For this review, take the finished solid that the model builds, in its own axes (mm). Coordinates: 2 decimals unless noted, no trailing zeros. Loops run counter-clockwise (first coordinate to the right, second up) from the corner with the lowest first, then second, coordinate; pieces in that order, holes last. Notation, with made-up numbers: (12.25, 74) -> (28.25, 74) arc R31 cw to (28.25, 105) -> close; hole circle Ø4 at (-27, 39.25). An arc over 180 degrees is marked (long way). Answer in a Markdown table with one row per item.
Autodesk Inventor part; units mm, degrees
ref_plane "YZ Plane" through (0, 0, 0) normal (1, 0, 0) x (0, 1, 0)
ref_plane "XZ Plane" through (0, 0, 0) normal (0, 1, 0) x (-1, 0, 0)
ref_plane "XY Plane" through (0, 0, 0) normal (0, 0, 1) x (1, 0, 0)
sketch "Sketch1" plane through (0, 0, 0) normal (0, 0, 1) x (1, 0, 0)
  circle A0 centre (0, 0) radius 12
  circle A1 centre (-6, 6) radius 2
  circle A2 centre (-6, -6) radius 2
  circle A3 centre (6, -6) radius 2
  circle A4 centre (6, 6) radius 2
  dimension "d0" = 24
  dimension "d1" = 4
  dimension "d2" = 6
  dimension "d3" = 6
  dimension "d6" = 360
extrude "Extrusion1" add sketch "Sketch1" along normal blind 6
sketch "Sketch2" plane through (0, 0, 6) normal (0, 0, 1) x (1, 0, 0)
  circle A0 centre (0, 0) radius 3.2
  dimension "d10" = 6.4
extrude "Extrusion2" cut sketch "Sketch2" against normal through all
properties part number "MountingPiece"
Item 1: Take a section at D-D, the plane z = 1.5. State the section outline as (x, y) points.
Worked answers:
| item | result |
|---|---|
| outline | circle Ø24 at (0, 0); hole circle Ø4 at (-6, -6); hole circle Ø4 at (-6, 6); hole circle Ø6.4 at (0, 0); hole circle Ø4 at (6, -6); hole circle Ø4 at (6, 6) |
Item 2: Insertion check: pin 1 (2 mm diameter, centred on x = -3.5, z = 2, fed in from +Y); pin 2 (4.5 mm diameter, centred on x = -6, y = 6, fed in from +Z); pin 3 (2 mm diameter, centred on x = -8, z = 2, fed in from +Y). Each pin has a flat end and moves straight along its axis. Give the tip position at first contact, or say it passes through.
Worked answers:
| item | result |
|---|---|
| pin 1 | y = 11.74 |
| pin 2 | z = 6 |
| pin 3 | y = 9.75 |
Item 3: The part is to be moulded in two halves that separate along X. For faces 1 (the cylindrical face through (4.4, 7.2, 3)), 2 (the flat face through (2.5, -2.5, 0)), 3 (the cylindrical face through (-7.6, 7.2, 3)), 4 (the cylindrical face through (-11.99, -0.53, 2.96)), say which applies: +X half, -X half, draft (parallel to the pull), parting line (faces both ways), or undercut.
Worked answers:
| item | result |
|---|---|
| face 1 | undercut |
| face 2 | draft |
| face 3 | undercut |
| face 4 | parting line |
Item 4: Take a section at C-C, the plane y = 6. State the section outline as (x, z) points.
Worked answers:
| item | result |
|---|---|
| outline | (-10.39, 0) -> (-8, 0) -> (-8, 6) -> (-10.39, 6) -> close; (-4, 0) -> (4, 0) -> (4, 6) -> (-4, 6) -> close; (8, 0) -> (10.39, 0) -> (10.39, 6) -> (8, 6) -> close |
Item 5: For L1, parallel to X at y = -4.75, z = 2.4; L2, parallel to X at y = 7, z = 3.5; L3, parallel to Y at x = 5, z = 5.05, list the stretches that pass through material, from the lowest coordinate up.
Worked answers:
| item | result |
|---|---|
| L1 | -11.02 to -7.56, -4.44 to 4.44, 7.56 to 11.02 |
| L2 | -9.75 to -7.73, -4.27 to 4.27, 7.73 to 9.75 |
| L3 | -10.91 to -7.73, -4.27 to 4.27, 7.73 to 10.91 |
Item 6: Take a section at A-A, the plane y = 0. State the section outline as (x, z) points.
Worked answers:
| item | result |
|---|---|
| outline | (-12, 0) -> (-3.2, 0) -> (-3.2, 6) -> (-12, 6) -> close; (3.2, 0) -> (12, 0) -> (12, 6) -> (3.2, 6) -> close |
